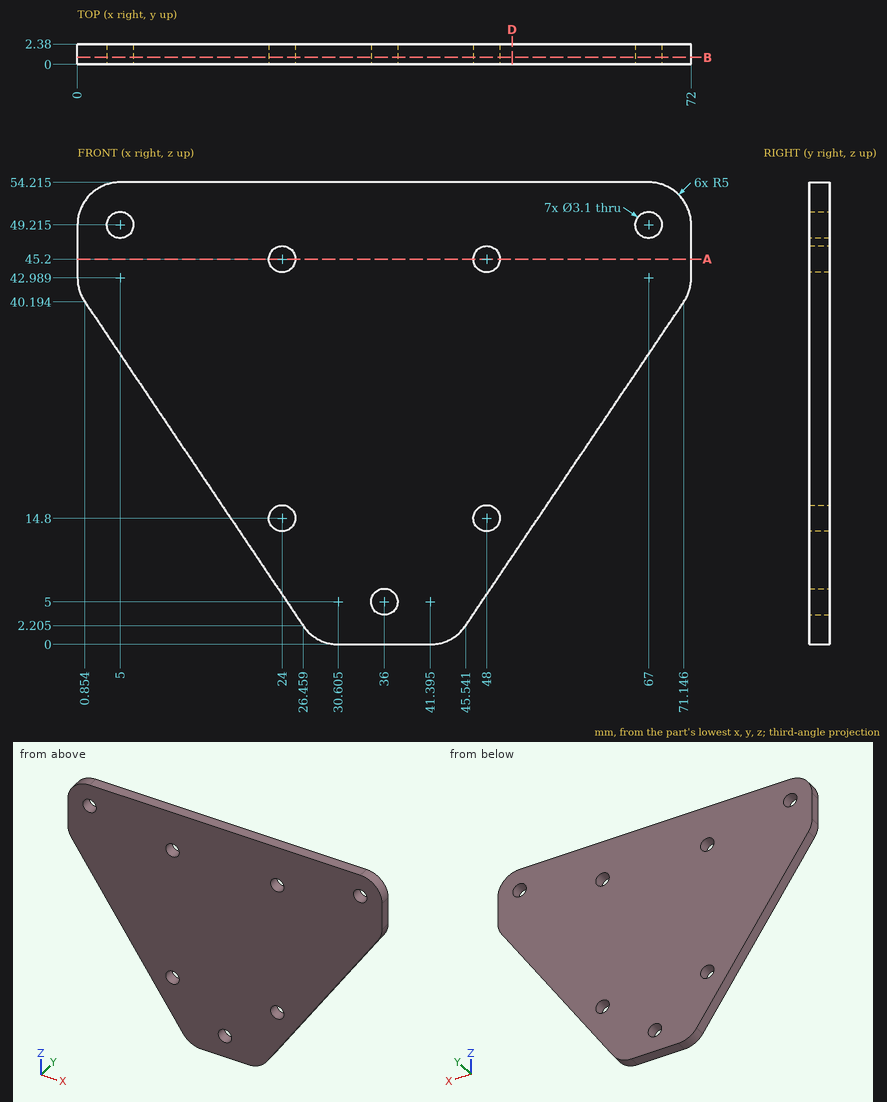
The drawing under review shows one solid part. Ordinate dimensions are in mm from its lowest x, y, z. Give positions to 0.01 mm unless a question says otherwise; leave off trailing zeros. Order: outer loops, then holes, each group sorted by start corner. A loop starts at its lowest first (then second) coordinate and runs counter-clockwise, first axis right, second up. Notation, with made-up numbers: (3.25, 6) - (29.25, 6) arc R32 cw to (29.25, 39) - close; hole circle Ø4 at (36.25, 72.5). An arc over 180 degrees is marked (long way). Answer as a JSON object with one key per item and string values. Group by question number.
Item 1: Clearance check with a flat-ended pin moving along its axis: pin 1 Ø1.9 at (x, z) = (24, 45.2) entering from -Y. State where the tip first meets the part, or that it passes through.
Item 2: Take a section at D-D on x = 51. Give the boundary of the cut face in (y, z) (1 decimal).
Item 3: Wall thickness on line 1 along X through (y, z) = (0.5, 45.2); line 2 along X through (y, z) = (1.1, 14.8); line 3 along Z through (x, y) = (67, 1.7) (1 decimal): over which ranges is each line inside the solid? List them lowest first.
Item 4: Take a section at B-B on y = 0.8. Give the number of separate pieces and of enclosed holes in the cut face, and give its area (3 significant figures).
Item 5: Take a section at A-A on z = 45.2. Give the boundary of the cut face in (x, y).
Reported:
{
 "1": {"pin 1": "through"},
 "2": {"outline": "(0, 10.3) - (2.4, 10.3) - (2.4, 54.2) - (0, 54.2) - close"},
 "3": {"line 1": "0 to 22.45, 25.55 to 46.45, 49.55 to 72", "line 2": "17.97 to 22.45, 25.55 to 46.45, 49.55 to 54.03", "line 3": "34 to 47.7, 50.8 to 54.2"},
 "4": {"separate pieces": "1", "enclosed holes": "7", "area": "2,680 mm^2"},
 "5": {"outline": "(0, 0) - (22.45, 0) - (22.45, 2.38) - (0, 2.38) - close; (25.55, 0) - (46.45, 0) - (46.45, 2.38) - (25.55, 2.38) - close; (49.55, 0) - (72, 0) - (72, 2.38) - (49.55, 2.38) - close"}
}
